The model under review builds one solid part; all positions refer to its coordinate system, in mm. A direction names the side the tool comes from. Round coordinates to 2 decimals unless told otherwise and drop trailing zeros. Write each loop counter-clockwise with the first axis right and the second up, starting at its lowest first coordinate (ties: lowest second). Pieces come first, ordered by that corner, then holes. Notation, with made-up numbers: M 57,87.25 L 73,87.25 A4 cw 73,94.25 Z; hole C 12.5,-1 d3. An arc over 180 degrees is marked long. One line per item, written item: value. Start each with the question number.
1) Take a section at B-B, the plane y = -10.5. Write out the cut boundary in (x, z), and give its area (3 significant figures).
2) Wall thickness on probe 1 along Y at (x, z) = (-16.6, 84.5); probe 2 along Z at (x, y) = (-16.65, -10.5); probe 3 along X at (y, z) = (5.75, 98): over which ranges is each line inside the solid? List them lowest first.
3) For P1, Ø6, axis at y = -3.5, z = 87.5, coming from the -X side; P2, Ø1.3, axis at x = -19, y = 1.5, coming from the +Z side; P3, Ø0.8, axis at x = -15, z = 85.5, coming from the +Y side, all flat-tipped, find the tip position at first contact; note any pin that passes through.
4) Take a section at D-D, the plane z = 87.5. Write out the cut boundary in (x, y).
5) Mouldability with a two-part tool opening along Z and no side actions: class faces 1 (the face through (-16.4, 10.5, 85.6)), 2 (the face through (-15, 0, 88)), 3 (the face through (-19, 4.25, 97)) as +Z half, -Z half, draft (parallel to the pull), parting line (faces both ways), or undercut.
6) Take a section at A-A, the plane z = 97. Write out the cut boundary in (x, y), and give its area (4 significant figures).
7) Tool access review of faces 4 (the face through (-19, 0, 92.75)), 5 (the face through (-19, -4.25, 97)), 6 (the face through (-19, 0, 101.25)): name each direction out of +Z, -Z, +X, -X, +Y, -Y from which nothing blocks a thin tool from reaching the whole face with its end or side.
8) Take a section at C-C, the plane y = -1. Write out the cut boundary in (x, z), and give its area (3 significant figures).
from build123d import *

# Parameters (mm, degrees)
CROQUIS1_W              = 23.86
CROQUIS1_H              = 25
SALIENTE_EXTRUIR1_DEPTH = 1
CROQUIS2_R              = 1.1
CORTAR_EXTRUIR1_DEPTH   = 3
CROQUIS3_W              = 8.5
CROQUIS3_H              = 8.5
SALIENTE_EXTRUIR2_DEPTH = 4.5
CROQUIS4_W              = 5.5
CROQUIS4_H              = 16
SALIENTE_EXTRUIR3_DEPTH = 2.5


with BuildPart() as part:
    # Croquis1 → Saliente-Extruir1 (new body)
    with BuildSketch(Plane(origin=(-16.9, 0, 0), x_dir=(0, 0, -1), z_dir=(1, 0, 0))):
        with Locations((-94.43, 0)):
            Rectangle(CROQUIS1_W, CROQUIS1_H)
    extrude(amount=SALIENTE_EXTRUIR1_DEPTH)

    # Croquis2 → Cortar-Extruir1 (cut)
    with BuildSketch(Plane(origin=(-17.9, 0, 0), x_dir=(0, 0, -1), z_dir=(1, 0, 0))):
        with Locations((-97, -10.5)):
            Circle(CROQUIS2_R)
        with Locations((-84.5, -10.5)):
            Circle(CROQUIS2_R)
        with Locations((-97, 10.5)):
            Circle(CROQUIS2_R)
        with Locations((-84.5, 10.5)):
            Circle(CROQUIS2_R)
    extrude(amount=CORTAR_EXTRUIR1_DEPTH, mode=Mode.SUBTRACT)

    # Croquis3 → Saliente-Extruir2 (add)
    with BuildSketch(Plane(origin=(-21.4, 0, 0), x_dir=(0, 0, -1), z_dir=(1, 0, 0))):
        with Locations((-97, 0)):
            Rectangle(CROQUIS3_W, CROQUIS3_H)
    extrude(amount=SALIENTE_EXTRUIR2_DEPTH)

    # Croquis4 → Saliente-Extruir3 (add)
    with BuildSketch(Plane(origin=(-15.9, 0, 0), x_dir=(0, 0, -1), z_dir=(1, 0, 0))):
        with Locations((-85.25, 0)):
            Rectangle(CROQUIS4_W, CROQUIS4_H)
    extrude(amount=SALIENTE_EXTRUIR3_DEPTH)


solid = part.part
Checked values:
1. outline: M -16.9,82.5 L -15.9,82.5 L -15.9,83.4 L -16.9,83.4 Z; M -16.9,85.6 L -15.9,85.6 L -15.9,95.9 L -16.9,95.9 Z; M -16.9,98.1 L -15.9,98.1 L -15.9,106.36 L -16.9,106.36 Z
1. area: 19.5 mm2
2. probe 1: y = -12.5 to -11.6, -9.4 to 9.4, 11.6 to 12.5
2. probe 2: z = 82.5 to 83.4, 85.6 to 95.9, 98.1 to 106.36
2. probe 3: x = -16.9 to -15.9
3. P1: stops at x = -16.9
3. P2: stops at z = 101.25
3. P3: stops at y = 8
4. outline: M -16.9,-12.5 L -15.9,-12.5 L -15.9,-8 L -13.4,-8 L -13.4,8 L -15.9,8 L -15.9,12.5 L -16.9,12.5 Z
5. face 1: undercut
5. face 2: +Z half
5. face 3: draft
6. outline: M -21.4,-4.25 L -16.9,-4.25 L -16.9,-9.4 L -15.9,-9.4 L -15.9,9.4 L -16.9,9.4 L -16.9,4.25 L -21.4,4.25 Z; M -16.9,-12.5 L -15.9,-12.5 L -15.9,-11.6 L -16.9,-11.6 Z; M -16.9,11.6 L -15.9,11.6 L -15.9,12.5 L -16.9,12.5 Z
6. area: 58.85 mm2
7. face 4: -Z, -X, +Y, -Y
7. face 5: +Z, -Z, -X, -Y
7. face 6: +Z, -X, +Y, -Y
8. outline: M -21.4,92.75 L -16.9,92.75 L -16.9,82.5 L -13.4,82.5 L -13.4,88 L -15.9,88 L -15.9,106.36 L -16.9,106.36 L -16.9,101.25 L -21.4,101.25 Z
8. area: 75.9 mm2
